```python
from build123d import *

# Parameters (mm, degrees)
F1_DEPTH = 12.7
F4_DEPTH = 6.35
F2_R     = 12.7
F5_DEPTH = 19.051
F2_R_2   = 6.35
F6_DEPTH = 6.35


with BuildPart() as f1:
    # F0 (on Top) → F1 (new body)
    with BuildSketch(Plane.XY):
        with BuildLine():
            Line((-38.1, -19.05), (0, -19.05))
            Line((0, -19.05), (0, -12.7))
            Line((0, -12.7), (25.4, -12.7))
            ThreePointArc((25.4, -12.7), (30.250968, 0), (25.4, 12.7))
            Line((25.4, 12.7), (0, 12.7))
            Line((0, 12.7), (0, 19.05))
            Line((0, 19.05), (-38.1, 19.05))
            ThreePointArc((-38.1, 19.05), (-57.15, 0), (-38.1, -19.05))
        make_face()
    extrude(amount=F1_DEPTH)

    # F3 (on face) → F4 (join)
    with BuildSketch(Plane(origin=(0, 0, 0), x_dir=(1, 0, 0), z_dir=(0, 0, -1))):
        with BuildLine():
            Line((12.91321, 25.4), (-37.88679, 25.4))
            ThreePointArc((-37.88679, 25.4), (-63.28679, 0), (-37.88679, -25.4))
            Line((-37.88679, -25.4), (12.91321, -25.4))
            ThreePointArc((12.91321, -25.4), (38.31321, 0), (12.91321, 25.4))
        make_face()
    extrude(amount=F4_DEPTH)

    # F2 (on face) → F5 (cut, through all)
    with BuildSketch(Plane.XY.offset(12.7)):
        with Locations((-38.1, 0)):
            Circle(F2_R)
    extrude(amount=-F5_DEPTH, mode=Mode.SUBTRACT)

    # F2 (on face) → F6 (join)
    with BuildSketch(Plane.XY.offset(12.7)):
        with Locations((6.35, 0)):
            Circle(F2_R_2)
    extrude(amount=F6_DEPTH)


solid = f1.part
```
Source: CAD feature listing. Evaluate the final solid. Frame: model axes, mm. A direction names the side the tool comes from. Give positions to 0.01 mm unless a question says otherwise; leave off trailing zeros. Loops run counter-clockwise (first coordinate to the right, second up) from the corner with the lowest first, then second, coordinate; pieces in that order, holes last. Notation, with made-up numbers: (3.25, 18) - (28.25, 18) arc R22 cw to (28.25, 53) - close; hole circle Ø7 at (-21, 44). An arc over 180 degrees is marked (long way). Use CSV: the item, a comma, the result in double quotes. Start each with the question number.
1. Reachability of faces 1 (the cylindrical face through (12.216, -2.432, 15.831)), 2 (the flat face through (0, -16, 6)), 3 (the flat face through (0, 16, 6)), 4 (the cylindrical face through (30.25, -0.19, 6.26)) from +Z, -Z, +X, -X, +Y, -Y: full face, straight path, thin tool, end or side. Return the list, or none.
2. Section D-D (y = -16.5). Output: boundary loops of the cut face in (x, z).
3. Pin query (flat end, axial travel): pin 1 (6.5 mm diameter, centred on x = 16, z = 5.5, fed in from +Y); pin 2 (1.5 mm diameter, centred on y = -16.5, z = 9, fed in from +X); pin 3 (4 mm diameter, centred on x = -47.5, z = 6.5, fed in from -Y). Return the tip coordinate at first contact, or that it passes through.
4. Section A-A (z = 5.5). Output: boundary loops of the cut face in (x, y).
5. Ray query, L1, parallel to Y at x = -38.1, z = 5.25; L2, parallel to Z at x = -49, y = 16; L3, parallel to Y at x = -21, z = 5.75. Return the intervals inside material, ascending.
6. Draft query along Y for faces 5 (the flat face through (-19, -19.05, 6)), 6 (the flat face through (13, 12.7, 6)), 7 (the cylindrical face through (-48.2, -7.7, 3.3)). Return one class per face: +Y half, -Y half, draft (parallel to the pull), parting line (faces both ways), or undercut.
7. Section C-C (x = 6.35). Output: boundary loops of the cut face in (y, z).
8. Section B-B (y = 0). Output: boundary loops of the cut face in (x, z).
Response:
1,face 1,"+Z"
1,face 2,"+Z, +X, -Y"
1,face 3,"+Z, +X, +Y"
1,face 4,"+Z, +X"
2,outline,"(-57.2, -6.35) - (32.22, -6.35) - (32.22, 0) - (0, 0) - (0, 12.7) - (-47.62, 12.7) - (-47.62, 0) - (-57.2, 0) - close"
3,pin 1,"y = 12.7"
3,pin 2,"x = 0"
3,pin 3,"y = -17.55"
4,outline,"(-38.1, -19.05) - (0, -19.05) - (0, -12.7) - (25.4, -12.7) arc R19.05 ccw to (25.4, 12.7) - (0, 12.7) - (0, 19.05) - (-38.1, 19.05) arc R19.05 ccw to start; hole circle Ø25.4 at (-38.1, 0)"
5,L1,"-19.05 to -12.7, 12.7 to 19.05"
5,L2,"-6.35 to 0"
5,L3,"-19.05 to 19.05"
6,face 5,"-Y half"
6,face 6,"+Y half"
6,face 7,"undercut"
7,outline,"(-25.4, -6.35) - (25.4, -6.35) - (25.4, 0) - (12.7, 0) - (12.7, 12.7) - (6.35, 12.7) - (6.35, 19.05) - (-6.35, 19.05) - (-6.35, 12.7) - (-12.7, 12.7) - (-12.7, 0) - (-25.4, 0) - close"
8,outline,"(-63.29, -6.35) - (-50.8, -6.35) - (-50.8, 12.7) - (-57.15, 12.7) - (-57.15, 0) - (-63.29, 0) - close; (-25.4, -6.35) - (38.31, -6.35) - (38.31, 0) - (30.25, 0) - (30.25, 12.7) - (12.7, 12.7) - (12.7, 19.05) - (0, 19.05) - (0, 12.7) - (-25.4, 12.7) - close"
